Part model, mm, in its own coordinate system. Round coordinates to 2 decimals unless told otherwise and drop trailing zeros. Loops run counter-clockwise (first coordinate to the right, second up) from the corner with the lowest first, then second, coordinate; pieces in that order, holes last. Notation, with made-up numbers: (23.5, 43) - (81.5, 43) arc R10 cw to (81.5, 61) - close; hole circle Ø9 at (37.25, -9.5). An arc over 180 degrees is marked (long way). Put each result on its own line as item: value.
from build123d import *

# Parameters (mm, degrees)
SKETCH1_R           = 30
BOSS_EXTRUDE1_DEPTH = 10
SKETCH2_R           = 3
CUT_EXTRUDE1_DEPTH  = 10
SKETCH4_R           = 4.318
SKETCH4_R_2         = 2.032
CUT_EXTRUDE2_DEPTH  = 10


with BuildPart() as part:
    # Sketch1 → Boss-Extrude1 (new body)
    with BuildSketch(Plane(origin=(0, 0, 0), x_dir=(1, 0, 0), z_dir=(0, 1, 0))):
        with Locations(Location((0, 0, 0), (0, 0, 270))):
            Circle(SKETCH1_R)
    extrude(amount=BOSS_EXTRUDE1_DEPTH)

    # Sketch2 → Cut-Extrude1 (cut)
    with BuildSketch(Plane(origin=(0, 10, 0), x_dir=(1, 0, 0), z_dir=(0, 1, 0))):
        with Locations(Location((0, -22, 0), (0, 0, 270))):
            Circle(SKETCH2_R)
        with Locations(Location((-19.052558883, -11, 0), (0, 0, 270))):
            Circle(SKETCH2_R)
        with Locations(Location((-19.052558883, 11, 0), (0, 0, 270))):
            Circle(SKETCH2_R)
        with Locations(Location((0, 22, 0), (0, 0, 270))):
            Circle(SKETCH2_R)
        with Locations(Location((19.052558883, 11, 0), (0, 0, 270))):
            Circle(SKETCH2_R)
        with Locations(Location((19.052558883, -11, 0), (0, 0, 270))):
            Circle(SKETCH2_R)
    extrude(amount=-CUT_EXTRUDE1_DEPTH, mode=Mode.SUBTRACT)

    # Sketch4 → Cut-Extrude2 (cut)
    with BuildSketch(Plane(origin=(0, 10, 0), x_dir=(1, 0, 0), z_dir=(0, 1, 0))):
        with Locations(Location((0, 0, 0), (0, 0, 270))):
            Circle(SKETCH4_R)
        with Locations(Location((0, -8.001, 0), (0, 0, 270))):
            Circle(SKETCH4_R_2)
        with Locations(Location((-8.001, 0, 0), (0, 0, 270))):
            Circle(SKETCH4_R_2)
        with Locations(Location((0, 8.001, 0), (0, 0, 270))):
            Circle(SKETCH4_R_2)
        with Locations(Location((8.001, 0, 0), (0, 0, 270))):
            Circle(SKETCH4_R_2)
    extrude(amount=-CUT_EXTRUDE2_DEPTH, mode=Mode.SUBTRACT)


solid = part.part
1. Pin check, flat tips, straight feed: P1, Ø3, axis at y = 5, z = 12, coming from the -X side; P2, Ø2, axis at x = 9.5, y = 4, coming from the +Z side; P3, Ø1.5, axis at y = 6, z = -11.5, coming from the +X side. Stop position of each tip, or through.
A:
P1: stops at x = -28.1
P2: stops at z = 28.77
P3: stops at x = 28.01
2. Band-saw the part on A-A (z = 0). List the corners of the cut face in (x, y).
A:
outline: (-30, 0) - (-10.03, 0) - (-10.03, 10) - (-30, 10) - close; (-5.97, 0) - (-4.32, 0) - (-4.32, 10) - (-5.97, 10) - close; (4.32, 0) - (5.97, 0) - (5.97, 10) - (4.32, 10) - close; (10.03, 0) - (30, 0) - (30, 10) - (10.03, 10) - close
3. Band-saw the part on D-D (y = 7). Give the number of separate pieces and of enclosed holes in the cut face, plus the area to 3 significant figures.
A:
separate pieces: 1
enclosed holes: 11
area: 2,550 mm²
4. Two-plate mould, pull along Z, no slides. Class faces 1 (the cylindrical face through (22.027, 5.07, -11.391)), 2 (the cylindrical face through (1.32, 4.93, -29.97)), 3 (the flat face through (-6, 10, 6)), 4 (the cylindrical face through (0, 5, 19)): pulls with the +Z half, pulls with the -Z half, needs draft (parallel to the pull), parting line crosses it, or undercut.
A:
face 1: undercut
face 2: parting line crosses it
face 3: needs draft
face 4: undercut
5. Band-saw the part on B-B (x = 0). List the corners of the cut face in (y, z), plus the area to 3 significant figures.
A:
outline: (0, -30) - (10, -30) - (10, -25) - (0, -25) - close; (0, -19) - (10, -19) - (10, -10.03) - (0, -10.03) - close; (0, -5.97) - (10, -5.97) - (10, -4.32) - (0, -4.32) - close; (0, 4.32) - (10, 4.32) - (10, 5.97) - (0, 5.97) - close; (0, 10.03) - (10, 10.03) - (10, 19) - (0, 19) - close; (0, 25) - (10, 25) - (10, 30) - (0, 30) - close
area: 312 mm²
6. Band-saw the part on C-C (z = 7). List the corners of the cut face in (x, y).
A:
outline: (-29.17, 0) - (-1.77, 0) - (-1.77, 10) - (-29.17, 10) - close; (1.77, 0) - (29.17, 0) - (29.17, 10) - (1.77, 10) - close
7. Probe line 1 along Z through (x, y) = (17, 4.25); line 2 along Z through (x, y) = (-19.5, 9.75); line 3 along Z through (x, y) = (1, 6.75). List the from-to ranges inside material, lowest first. Write a range as [from, to].
A:
line 1: z = [-24.72, -13.19], [-8.81, 8.81], [13.19, 24.72]
line 2: z = [-22.8, -13.97], [-8.03, 8.03], [13.97, 22.8]
line 3: z = [-29.98, -24.83], [-19.17, -9.77], [-6.23, -4.2], [4.2, 6.23], [9.77, 19.17], [24.83, 29.98]
